Part print with two shaded views. Sizes in mm from the minimum x, y, z corner. A direction names the side the tool comes from. Round coordinates to 2 decimals unless told otherwise and drop trailing zeros. Loops run counter-clockwise (first coordinate to the right, second up) from the corner with the lowest first, then second, coordinate; pieces in that order, holes last. Notation, with made-up numbers: (-5.75, 61.25) - (50.25, 61.25) arc R25 cw to (50.25, 98.25) - close; hole circle Ø1 at (3, 24.5). An arc over 180 degrees is marked (long way). Put each result on its own line as item: value. Start each with the question number.
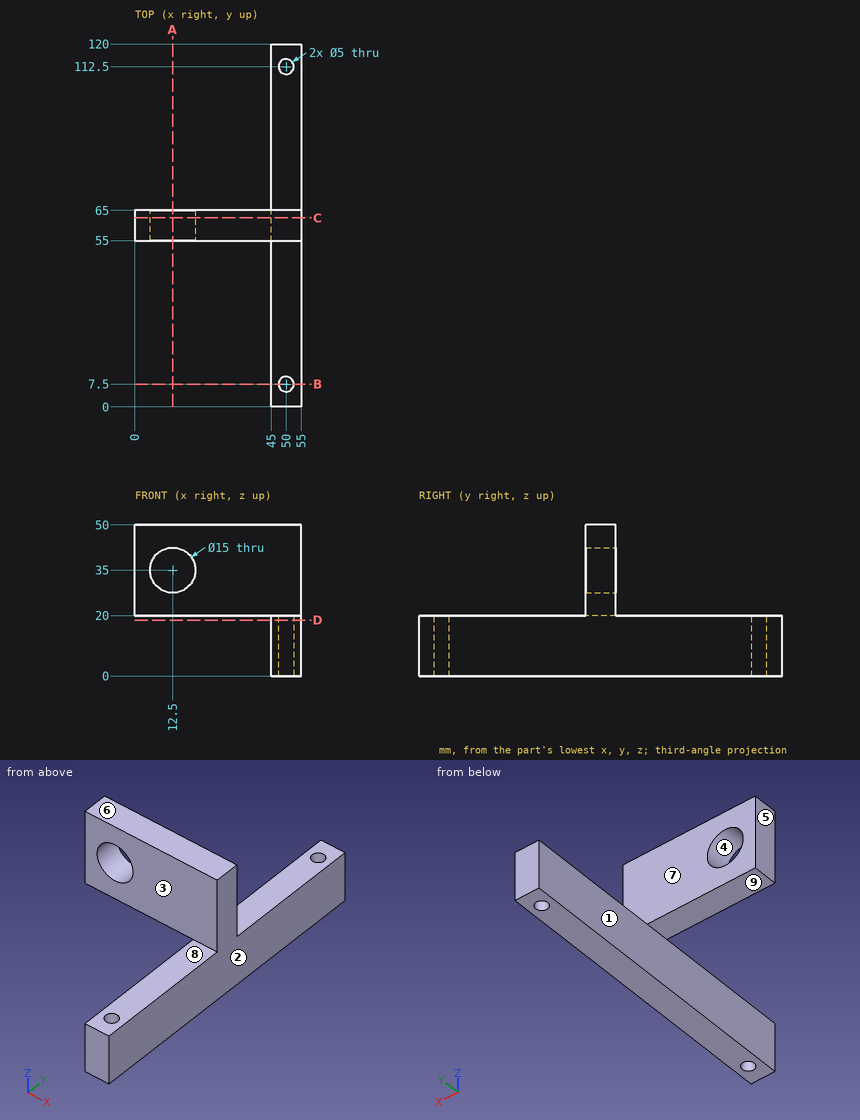
1) Which spindle directions (+Z, -Z, +X, -X, +Y, -Y) get a long thin tool onto all of the face, cutting with end or side? Do the marked faces 5, 6, 7, 8 and 9. Say none if no direction does.
2) Slice it at A-A, the plane x = 12.5. Write the cut outline in (y, z), and give its area (3 significant figures).
3) Slice it at B-B, the plane y = 7.5. Write the cut outline in (x, z), and give its area (3 significant figures).
4) Drop flat-ended pins along their axis: pin 1 Ø19.5 at (x, z) = (12.5, 35) entering from -Y; pin 2 Ø11 at (x, y) = (21.5, 59) entering from -Z; pin 3 Ø2 at (x, z) = (7, 27) entering from +Y; pin 4 Ø3 at (x, y) = (43, 46.5) entering from -Z. Give the stop position or say it passes through.
5) Pull direction X, two halves, no side cores. Call the marked faces 1, 2, 3 and 4: pulls with the +X half, pulls with the -X half, needs draft (parallel to the pull), parting line crosses it, or undercut.
6) Slice it at C-C, the plane y = 62.5. Write the cut outline in (x, z).
7) Drill centre lines: line 1 (Y direction, x = 50, z = 4.75); line 2 (Z direction, x = 12.5, y = 59); line 3 (Y direction, x = 31, z = 29). Where is each one in solid material? Low to high. Write a range as [from, to].
8) Slice it at D-D, the plane z = 18.5. Write the cut outline in (x, y).
Taken from the geometry:
1. face 5: +Z, -Z, -X, +Y, -Y
1. face 6: +Z, +X, -X, +Y, -Y
1. face 7: +Z, +X, -X, +Y
1. face 8: +Z, +X, -X, -Y
1. face 9: -Z, -X, +Y, -Y
2. outline: (55, 20) - (65, 20) - (65, 27.5) - (55, 27.5) - close; (55, 42.5) - (65, 42.5) - (65, 50) - (55, 50) - close
2. area: 150 mm2
3. outline: (45, 0) - (47.5, 0) - (47.5, 20) - (45, 20) - close; (52.5, 0) - (55, 0) - (55, 20) - (52.5, 20) - close
3. area: 100 mm2
4. pin 1: stops at y = 55
4. pin 2: stops at z = 20
4. pin 3: stops at y = 65
4. pin 4: passes through
5. face 1: pulls with the -X half
5. face 2: pulls with the +X half
5. face 3: needs draft
5. face 4: undercut
6. outline: (0, 20) - (45, 20) - (45, 0) - (55, 0) - (55, 50) - (0, 50) - close; hole circle Ø15 at (12.5, 35)
7. line 1: y = [0, 5], [10, 110], [115, 120]
7. line 2: z = [20, 27.5], [42.5, 50]
7. line 3: y = [55, 65]
8. outline: (45, 0) - (55, 0) - (55, 120) - (45, 120) - close; hole circle Ø5 at (50, 7.5); hole circle Ø5 at (50, 112.5)
